For this review, use the dimensioned drawing (mm, ordinates from the lowest corner) and the shaded views. Round coordinates to 2 decimals unless told otherwise and drop trailing zeros. Write each loop counter-clockwise with the first axis right and the second up, starting at its lowest first coordinate (ties: lowest second). Pieces come first, ordered by that corner, then holes.
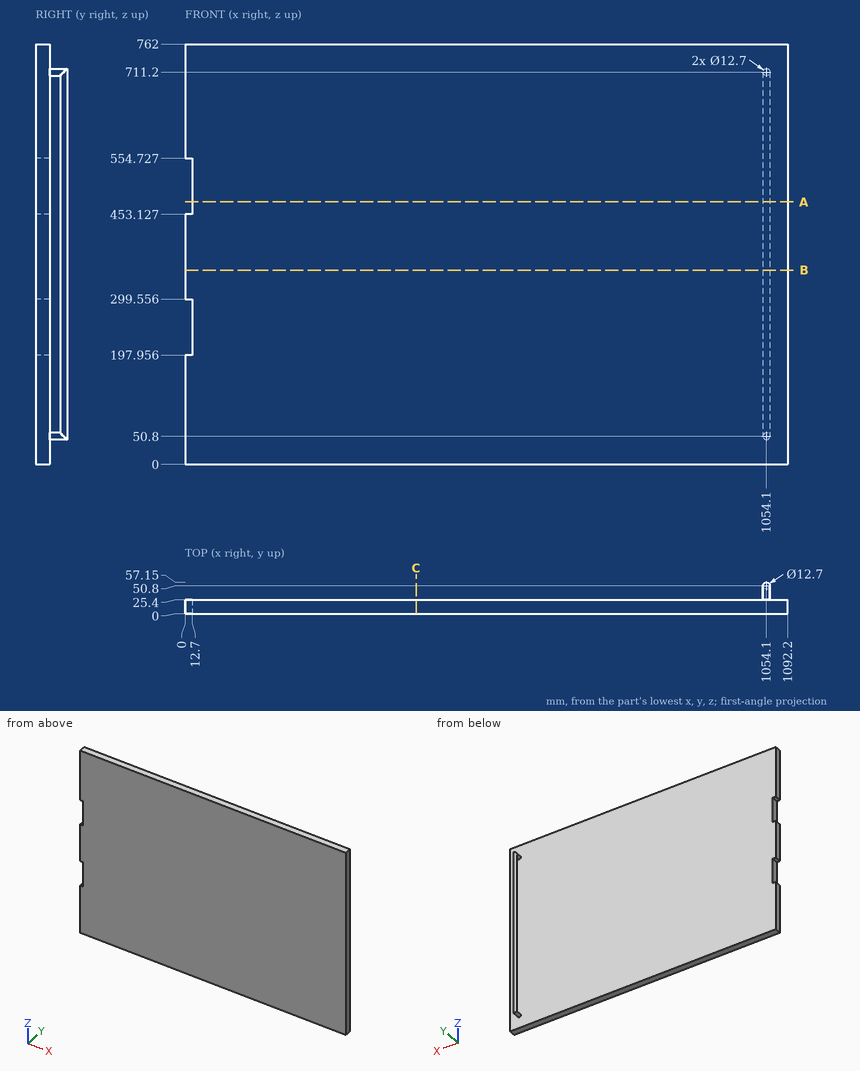
(1) For pin 1 Ø6 at (x, z) = (457, 296.5) entering from +Y; pin 2 Ø7.5 at (y, z) = (14, 526.5) entering from -X; pin 3 Ø2 at (y, z) = (45.5, 148.5) entering from +X, all flat-tipped, find the tip position at first contact; note any pin that passes through.
Geometry check:
pin 1: stops at y = 25.4
pin 2: stops at x = 12.7
pin 3: stops at x = 1058.77
(2) We need section C-C, the plane x = 419. Give the boundary of the cut face in (y, z), and give its area (3 significant figures).
Geometry check:
outline: (0, 0) - (25.4, 0) - (25.4, 762) - (0, 762) - close
area: 19,400 mm2
(3) We need section B-B, the plane z = 352. Give the boundary of the cut face in (x, y).
Geometry check:
outline: (0, 0) - (1092.2, 0) - (1092.2, 25.4) - (0, 25.4) - close; circle Ø12.7 at (1054.1, 50.8)
(4) For line 1 along Y through (x, z) = (848, 536); line 2 along X through (y, z) = (10.5, 541); line 3 along X through (y, z) = (49, 643.5), list the stretches that pass through material, from the lowest coordinate up.
Geometry check:
line 1: y = 0 to 25.4
line 2: x = 12.7 to 1092.2
line 3: x = 1048.01 to 1060.19
(5) We need section A-A, the plane z = 476. Give the boundary of the cut face in (x, y), and give its area (3 significant figures).
Geometry check:
outline: (12.7, 0) - (1092.2, 0) - (1092.2, 25.4) - (12.7, 25.4) - close; circle Ø12.7 at (1054.1, 50.8)
area: 27,500 mm2
